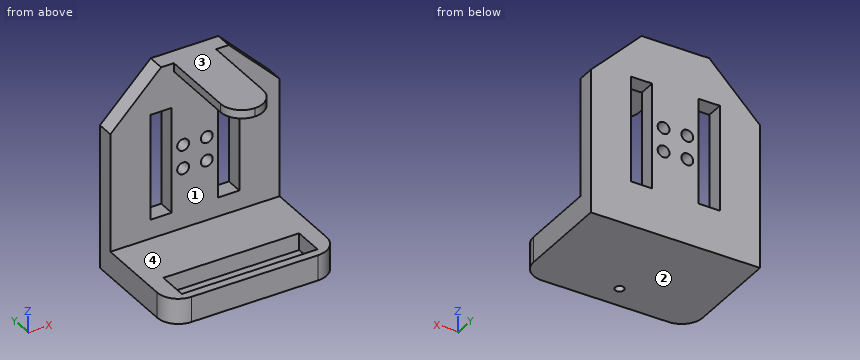
```python
from build123d import *

# Parameters (mm, degrees)
SCHIZZO3_W                   = 40
SCHIZZO3_H                   = 27
ESTRUSIONE_ESTRUSIONE1_DEPTH = 6
SCHIZZO4_W                   = 32.1
SCHIZZO4_H                   = 7.1
TAGLIO_ESTRUSIONE1_DEPTH     = 4
SCHIZZO5_R                   = 1.05
TAGLIO_ESTRUSIONE2_DEPTH     = 25.459149617
SCHIZZO6_W                   = 40
SCHIZZO6_H                   = 4
ESTRUSIONE_ESTRUSIONE2_DEPTH = 40
SCHIZZO7_W                   = 10
SCHIZZO7_H                   = 2
ESTRUSIONE_ESTRUSIONE3_DEPTH = 23
SCHIZZO8_R                   = 1.4
SCHIZZO8_W                   = 5
SCHIZZO8_H                   = 25
TAGLIO_ESTRUSIONE3_DEPTH     = 57.964901475
RACCORDO1_R                  = 5


with BuildPart() as part:
    # Schizzo3 → Estrusione-Estrusione1 (new body)
    with BuildSketch(Plane.XY):
        Rectangle(SCHIZZO3_W, SCHIZZO3_H)
    extrude(amount=ESTRUSIONE_ESTRUSIONE1_DEPTH)

    # Schizzo4 → Taglio-Estrusione1 (cut)
    with BuildSketch(Plane.XY.offset(6)):
        with Locations((0, -8)):
            Rectangle(SCHIZZO4_W, SCHIZZO4_H)
    extrude(amount=-TAGLIO_ESTRUSIONE1_DEPTH, mode=Mode.SUBTRACT)

    # Schizzo5 → Taglio-Estrusione2 (cut, through all)
    with BuildSketch(Plane.XY.offset(2)):
        with Locations((0, -8)):
            Circle(SCHIZZO5_R)
    extrude(amount=-TAGLIO_ESTRUSIONE2_DEPTH, mode=Mode.SUBTRACT)

    # Schizzo6 → Estrusione-Estrusione2 (add)
    with BuildSketch(Plane.XY.offset(6)):
        with Locations((0, 11.5)):
            Rectangle(SCHIZZO6_W, SCHIZZO6_H)
    extrude(amount=ESTRUSIONE_ESTRUSIONE2_DEPTH)

    # Schizzo7 → Estrusione-Estrusione3 (add)
    with BuildSketch(Plane.XZ.offset(-9.5)):
        with Locations((0, 45)):
            Rectangle(SCHIZZO7_W, SCHIZZO7_H)
    extrude(amount=ESTRUSIONE_ESTRUSIONE3_DEPTH)

    # Schizzo8 → Taglio-Estrusione3 (cut, through all)
    with BuildSketch(Plane(origin=(0, 13.5, 0), x_dir=(1, 0, 0), z_dir=(0, 1, 0))):
        with Locations(Location((-2.8, -20.2, 0), (0, 0, 270))):
            Circle(SCHIZZO8_R)
        with Locations(Location((-2.8, -25.8, 0), (0, 0, 270))):
            Circle(SCHIZZO8_R)
        with Locations(Location((2.8, -25.8, 0), (0, 0, 270))):
            Circle(SCHIZZO8_R)
        with Locations(Location((2.8, -20.2, 0), (0, 0, 270))):
            Circle(SCHIZZO8_R)
        with Locations((8, -23)):
            Rectangle(SCHIZZO8_W, SCHIZZO8_H)
        with Locations((-8, -23)):
            Rectangle(SCHIZZO8_W, SCHIZZO8_H)
        Polygon((-20, -34), (-8, -46), (-20, -46), align=None)
        Polygon((8, -46), (20, -46), (20, -34), align=None)
    extrude(amount=-TAGLIO_ESTRUSIONE3_DEPTH, mode=Mode.SUBTRACT)

    # Raccordo1
    raccordo1_edges = [part.edges().sort_by_distance(p)[0] for p in [
        (-5, -13.5, 45),
        (5, -13.5, 45),
        (20, -13.5, 3),
        (-20, -13.5, 3),
    ]]
    fillet(raccordo1_edges, radius=RACCORDO1_R - 0.0001)  # a hair under: the kernel refuses the full size


solid = part.part
```
The listing builds one solid part. Answer for the finished solid, in the listing's coordinates (mm). Face numbers are marked on the shaded views. Round coordinates to 2 decimals unless told otherwise and drop trailing zeros. Loops run counter-clockwise (first coordinate to the right, second up) from the corner with the lowest first, then second, coordinate; pieces in that order, holes last. Notation, with made-up numbers: (-6, 15.25) - (8, 15.25) arc R38 cw to (8, 53.25) - close; hole circle Ø3 at (-39.5, 27). An arc over 180 degrees is marked (long way). Use one line per item in the form item = value. Start each with the question number.
1. The part is cut by section B-B on y = 4.75. Determine the outline of the cut face in (x, z).
2. The part is cut by section D-D on z = 15. Determine the outline of the cut face in (x, y), then the cut area to 3 significant figures.
3. For a pull along Z with two mould halves and no side action, classify the marked faces 1, 2, 3 and 4 as pulls with the +Z half, pulls with the -Z half, needs draft (parallel to the pull), parting line crosses it, or undercut.
4. Given pin 1 Ø8 at (x, z) = (-8, 39.5) entering from -Y; pin 2 Ø1 at (x, y) = (9.5, 3.5) entering from +Z; pin 3 Ø1.6 at (y, z) = (3, 44.5) entering from -X, each flat-ended and moving along its own axis, determine where each tip first touches the part or whether it passes through.
5. Consider line 1 (Z direction, x = -4, y = -11.25); line 2 (Z direction, x = -13.5, y = -8.5); line 3 (Y direction, x = 17, z = 23). Determine where each line is inside the solid, lowest interval first. Write a range as [from, to].
6. The part is cut by section C-C on x = -9. Determine the outline of the cut face in (y, z), then the cut area to 3 significant figures.
7. The part is cut by section A-A on z = 20.2. Determine the outline of the cut face in (x, y), then the cut area to 3 significant figures.
Geometry check:
q1.outline = (-20, 0) - (20, 0) - (20, 6) - (-20, 6) - close; (-5, 44) - (5, 44) - (5, 46) - (-5, 46) - close
q2.outline = (-20, 9.5) - (-10.5, 9.5) - (-10.5, 13.5) - (-20, 13.5) - close; (-5.5, 9.5) - (5.5, 9.5) - (5.5, 13.5) - (-5.5, 13.5) - close; (10.5, 9.5) - (20, 9.5) - (20, 13.5) - (10.5, 13.5) - close
q2.area = 120 mm^2
q3.face_1 = undercut
q3.face_2 = pulls with the -Z half
q3.face_3 = pulls with the +Z half
q3.face_4 = undercut
q4.pin_1 = 9.5
q4.pin_2 = 6
q4.pin_3 = -5
q5.line_1 = [0, 2], [44, 46]
q5.line_2 = [0, 2]
q5.line_3 = [9.5, 13.5]
q6.outline = (-13.5, 0) - (13.5, 0) - (13.5, 10.5) - (9.5, 10.5) - (9.5, 6) - (-4.45, 6) - (-4.45, 2) - (-11.55, 2) - (-11.55, 6) - (-13.5, 6) - close; (9.5, 35.5) - (13.5, 35.5) - (13.5, 45) - (9.5, 45) - close
q6.area = 190 mm^2
q7.outline = (-20, 9.5) - (-10.5, 9.5) - (-10.5, 13.5) - (-20, 13.5) - close; (-5.5, 9.5) - (-4.2, 9.5) - (-4.2, 13.5) - (-5.5, 13.5) - close; (-1.4, 9.5) - (1.4, 9.5) - (1.4, 13.5) - (-1.4, 13.5) - close; (4.2, 9.5) - (5.5, 9.5) - (5.5, 13.5) - (4.2, 13.5) - close; (10.5, 9.5) - (20, 9.5) - (20, 13.5) - (10.5, 13.5) - close
q7.area = 97.6 mm^2
